Design review of the part built by this model. Coordinates are the model's own, in mm. Coordinates: 2 decimals unless noted, no trailing zeros. Loops run counter-clockwise (first coordinate to the right, second up) from the corner with the lowest first, then second, coordinate; pieces in that order, holes last. Notation, with made-up numbers: (56.5, 49) -> (96.5, 49) arc R33 cw to (96.5, 88) -> close; hole circle Ø8 at (0, -15). An arc over 180 degrees is marked (long way). Use a Markdown table: item, result. Add a question column.
Q1. For probe 1 along Z at (x, y) = (2.75, 44.5), list the stretches that pass through material, from the lowest coordinate up.
Q2. Clearance check with flat-ended pins moving along their axes: pin 1 Ø4 at (y, z) = (59, -130.5) entering from -X; pin 2 Ø3 at (x, y) = (2.5, 33.5) entering from +Z; pin 3 Ø1.9 at (x, y) = (4, 80.5) entering from -Z. State where each tip first meets the part, or that it passes through.
Q3. Take a section at B-B on y = 66.5. Write out the cut boundary in (x, z).
Q4. Take a section at A-A on x = 2. Write out the cut boundary in (y, z), plus the area to 3 significant figures.
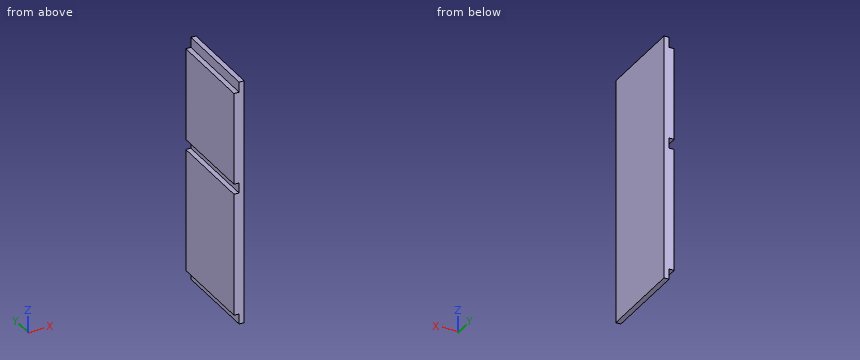
from build123d import *

# Parameters (mm, degrees)
SKETCH1_W           = 304.8
SKETCH1_H           = 114.3
BOSS_EXTRUDE1_DEPTH = 12.7
SKETCH2_W           = 12.7
SKETCH2_H           = 114.3
CUT_EXTRUDE1_DEPTH  = 6.35


with BuildPart() as part:
    # Sketch1 → Boss-Extrude1 (new body)
    with BuildSketch(Plane(origin=(0, 0, 0), x_dir=(0, 0, -1), z_dir=(1, 0, 0))):
        with Locations((152.4, 57.15)):
            Rectangle(SKETCH1_W, SKETCH1_H)
    extrude(amount=BOSS_EXTRUDE1_DEPTH)

    # Sketch2 → Cut-Extrude1 (cut)
    with BuildSketch(Plane.ZY):
        with Locations((-6.35, 57.15)):
            Rectangle(SKETCH2_W, SKETCH2_H)
        with Locations((-298.45, 57.15)):
            Rectangle(SKETCH2_W, SKETCH2_H)
        with Locations((-133.35, 57.15)):
            Rectangle(SKETCH2_W, SKETCH2_H)
    extrude(amount=-CUT_EXTRUDE1_DEPTH, mode=Mode.SUBTRACT)


solid = part.part
Answer list:
| question | item | result |
|---|---|---|
| 1 | probe 1 | -292.1 to -139.7, -127 to -12.7 |
| 2 | pin 1 | x = 6.35 |
| 2 | pin 2 | z = -12.7 |
| 2 | pin 3 | z = -292.1 |
| 3 | outline | (0, -292.1) -> (6.35, -292.1) -> (6.35, -304.8) -> (12.7, -304.8) -> (12.7, 0) -> (6.35, 0) -> (6.35, -12.7) -> (0, -12.7) -> (0, -127) -> (6.35, -127) -> (6.35, -139.7) -> (0, -139.7) -> close |
| 4 | outline | (0, -292.1) -> (114.3, -292.1) -> (114.3, -139.7) -> (0, -139.7) -> close; (0, -127) -> (114.3, -127) -> (114.3, -12.7) -> (0, -12.7) -> close |
| 4 | area | 30,500 mm² |
